```python
from build123d import *

# Parameters (mm, degrees)
SKETCH1_W          = 89.8724
SKETCH1_H          = 227.2896
SKETCH1_R          = 2
BODY_DEPTH         = 0.06858
SKETCH2_W          = 89.8724
SKETCH2_H          = 0.0686
TOP_OVERWRAP_DEPTH = 0.2896


with BuildPart() as part:
    # Sketch1 → Body (new body)
    with BuildSketch(Plane.XY):
        with Locations((-44.9362, 0)):
            Rectangle(SKETCH1_W, SKETCH1_H)
        with Locations((-83.71996894, -56.66618171)):
            Circle(SKETCH1_R, mode=Mode.SUBTRACT)
        with Locations((-83.71996894, 56.98616943)):
            Circle(SKETCH1_R, mode=Mode.SUBTRACT)
    body = extrude(amount=BODY_DEPTH)

    # Sketch2 → Top Overwrap (add)
    with BuildSketch(Plane(origin=(0, 227.3734, 0.06858), x_dir=(-1, 0, 0), z_dir=(0, 0, 1))):
        with Locations((44.9362, 113.7629)):
            Rectangle(SKETCH2_W, SKETCH2_H)
    top_overwrap = extrude(amount=TOP_OVERWRAP_DEPTH)

    # Mirror1: Body, Top Overwrap across plane
    add(body.mirror(Plane(origin=(0, 0, 0), x_dir=(0, 0, 1), z_dir=(1, 0, 0))))
    add(top_overwrap.mirror(Plane(origin=(0, 0, 0), x_dir=(0, 0, 1), z_dir=(1, 0, 0))))


solid = part.part
```
Here's how the part is built. I have some questions about the finished solid (model axes, mm). Give positions to 0.01 mm unless a question says otherwise; leave off trailing zeros. Write each loop counter-clockwise with the first axis right and the second up, starting at its lowest first coordinate (ties: lowest second). Pieces come first, ordered by that corner, then holes. Notation, with made-up numbers: (6.25, -20.75) -> (16.25, -20.75) arc R29 cw to (16.25, 9.25) -> close; hole circle Ø4 at (66, -15.5). An arc over 180 degrees is marked (long way). Use one line per item in the form item = value.
1) Suppose I cut it at A-A (x = -21.5). Please give me the cut outline in (y, z).
Verdict:
outline = (-113.64, 0) -> (113.64, 0) -> (113.64, 0.36) -> (113.58, 0.36) -> (113.58, 0.07) -> (-113.64, 0.07) -> close
2) Suppose I cut it at C-C (y = -92.5). Please give me the cut outline in (x, z), and give its area (3 significant figures).
Verdict:
outline = (-89.87, 0) -> (89.87, 0) -> (89.87, 0.07) -> (-89.87, 0.07) -> close
area = 12.3 mm2
3) I'm going to push flat-ended pins straight in: pin 1 (3 mm diameter, centred on x = -83.72, y = -56.67, fed in from +Z); pin 2 (4.5 mm diameter, centred on x = 83.72, y = 56.99, fed in from +Z). Where does each tip first touch, or does it pass through?
Verdict:
pin_1 = through
pin_2 = 0.07
4) Suppose I cut it at B-B (z = 0.2). Please give me the cut outline in (x, y), and give its area (3 significant figures).
Verdict:
outline = (-89.87, 113.58) -> (89.87, 113.58) -> (89.87, 113.64) -> (-89.87, 113.64) -> close
area = 12.3 mm2
